Can you work these out from the model? Positions are in its coordinate system, mm. A direction names the side the tool comes from. Give positions to 0.01 mm unless a question says otherwise; leave off trailing zeros. Write each loop counter-clockwise with the first axis right and the second up, starting at its lowest first coordinate (ties: lowest second). Pieces come first, ordered by that corner, then holes.
from build123d import *

# Parameters (mm, degrees)
SKETCH1_W           = 15.5
SKETCH1_H           = 12.8
BOSS_EXTRUDE1_DEPTH = 4.5
SKETCH2_R           = 1
BOSS_EXTRUDE2_DEPTH = 4
BOSS_EXTRUDE3_DEPTH = 2


with BuildPart() as part:
    # Sketch1 → Boss-Extrude1 (new body)
    with BuildSketch(Plane.XY):
        Rectangle(SKETCH1_W, SKETCH1_H)
    extrude(amount=BOSS_EXTRUDE1_DEPTH)

    # Sketch2 → Boss-Extrude2 (add)
    with BuildSketch(Plane(origin=(0, 0, 0), x_dir=(1, 0, 0), z_dir=(0, 0, -1))):
        with Locations(Location((0, 0, 0), (0, 0, 270))):
            Circle(SKETCH2_R)
    extrude(amount=BOSS_EXTRUDE2_DEPTH)

    # Sketch3 → Boss-Extrude3 (add)
    with BuildSketch(Plane.XY.offset(4.5)):
        Polygon((-7.75, 2), (-8.75, 2), (-8.75, -2), (-7.75, -2), (7.75, -2), (8.75, -2), (8.75, 2), (7.75, 2), align=None)
    extrude(amount=BOSS_EXTRUDE3_DEPTH)


solid = part.part
(1) Imagine slicing it at A-A, the plane x = 4.25. Write out the boundary of the cut face in (y, z).
Returned:
outline: (-6.4, 0) - (6.4, 0) - (6.4, 4.5) - (2, 4.5) - (2, 6.5) - (-2, 6.5) - (-2, 4.5) - (-6.4, 4.5) - close
(2) Will these pins go through, and if not, where does the flat tip stop? P1, Ø2, axis at x = 3.5, y = -0.5, coming from the -Z side; P2, Ø3.5, axis at y = 3, z = 2, coming from the -X side; P3, Ø1.3, axis at x = -1, y = 3, coming from the +Z side.
Returned:
P1: stops at z = 0
P2: stops at x = -7.75
P3: stops at z = 4.5
(3) Imagine slicing it at B-B, the plane y = 0. Write out the boundary of the cut face in (x, z), plus the area to 3 significant figures.
Returned:
outline: (-8.75, 4.5) - (-7.75, 4.5) - (-7.75, 0) - (-1, 0) - (-1, -4) - (1, -4) - (1, 0) - (7.75, 0) - (7.75, 4.5) - (8.75, 4.5) - (8.75, 6.5) - (-8.75, 6.5) - close
area: 113 mm2
(4) Imagine slicing it at D-D, the plane x = 0. Write out the boundary of the cut face in (y, z), plus the area to 3 significant figures.
Returned:
outline: (-6.4, 0) - (-1, 0) - (-1, -4) - (1, -4) - (1, 0) - (6.4, 0) - (6.4, 4.5) - (2, 4.5) - (2, 6.5) - (-2, 6.5) - (-2, 4.5) - (-6.4, 4.5) - close
area: 73.6 mm2
(5) If I drill on L1, parallel to Y at x = -3.5, z = 5.5; L2, parallel to Z at x = -2.5, y = -1; L3, parallel to Z at x = 3.5, y = -4.25, over which ranges is the centre line in solid material (lowest first)?
Returned:
L1: y = -2 to 2
L2: z = 0 to 6.5
L3: z = 0 to 4.5
(6) For faces 1 (the face through (7.75, 0, 2)), 2 (the face through (-8, 0, 4.5)), 3 (the face through (0, 4, 4.5)), which set-ups out of +Z, -Z, +X, -X, +Y, -Y let a thin tool reach every point of the face, with its end or its side?
Returned:
face 1: -Z, +X, +Y, -Y
face 2: -Z, -X, +Y, -Y
face 3: +Z, +X, -X, +Y
(7) Imagine slicing it at C-C, the plane z = -0.25. Write out the boundary of the cut face in (x, y), plus the area to 3 significant figures.
Returned:
outline: circle Ø2 at (0, 0)
area: 3.14 mm2
